Geometry check sheet. Reference: drawing and pictorial views, mm from the part's lowest x, y, z. A direction names the side the tool comes from. Round coordinates to 2 decimals unless told otherwise and drop trailing zeros. Order: outer loops, then holes, each group sorted by start corner. A loop starts at its lowest first (then second) coordinate and runs counter-clockwise, first axis right, second up.
(1) Go/stop test with flat-tipped pins: pin 1 (5 mm diameter, centred on y = 2.5, z = 6, fed in from +X); pin 2 (1.6 mm diameter, centred on x = 7, z = 4.5, fed in from +Y); pin 3 (3 mm diameter, centred on x = 11.5, y = 7, fed in from +Z). Record where each tip stops, or that it passes through.
(2) Sectioned sample at C-C (y = 6.5). Record the boundary of the cut face in (x, z), plus the area to 3 significant figures.
(3) Release check for a two-part mould opening along X. For the marked faces 3, 4 and 5 record: +X half, -X half, draft (parallel to the pull), parting line (faces both ways), or undercut.
(4) Material ranges on line 1 along X through (y, z) = (10.5, 6); line 2 along Y through (x, z) = (7, 6); line 3 along Y through (x, z) = (6.5, 12.5), recorded low to high.
(5) Sectioned sample at B-B (x = 4.75). Record the boundary of the cut face in (y, z).
(6) Sectioned sample at A-A (z = 7). Record the boundary of the cut face in (x, y).
(7) Sectioned sample at D-D (z = 8.75). Record the boundary of the cut face in (x, y), plus the area to 3 significant figures.
(8) Set-up check for the marked faces 1 and 2: record each of +Z, -Z, +X, -X, +Y, -Y from which the full face is reachable in a straight line by a thin tool's end or side.
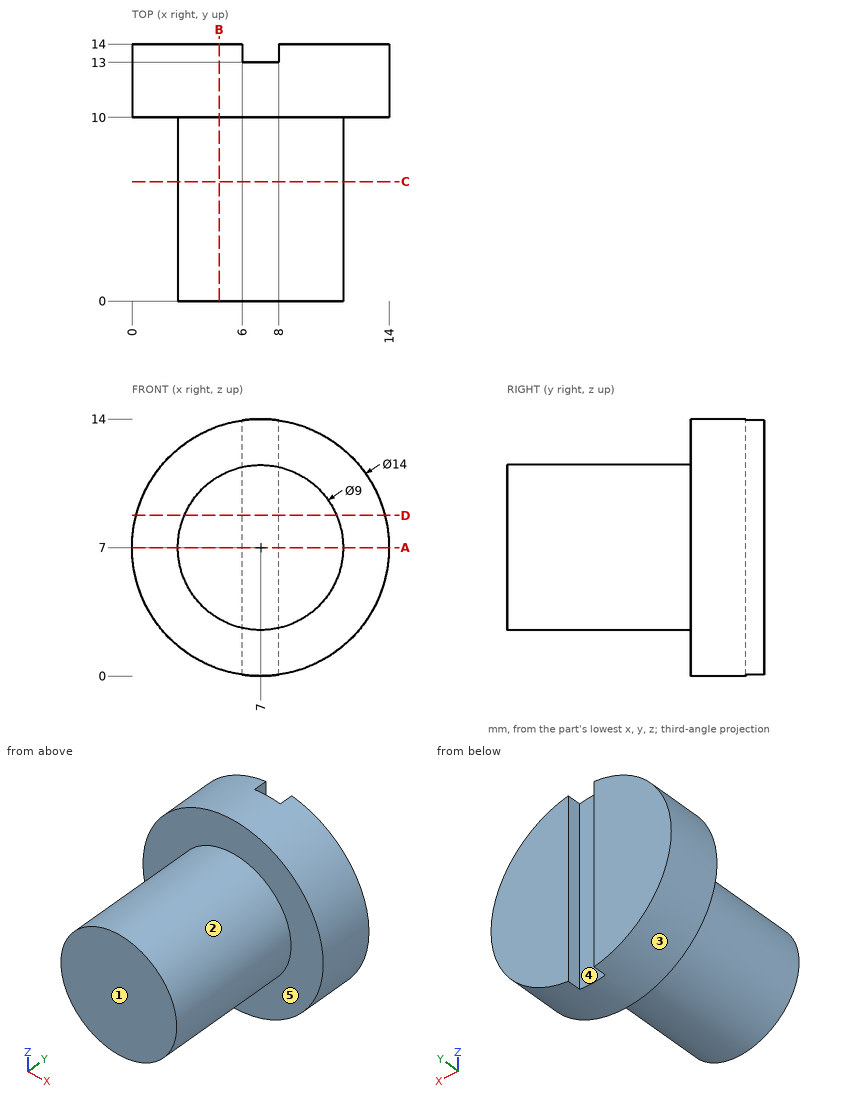
Answer below:
1. pin 1: stops at x = 11.5
1. pin 2: stops at y = 13
1. pin 3: stops at z = 10.35
2. outline: circle Ø9 at (7, 7)
2. area: 63.6 mm2
3. face 3: parting line
3. face 4: undercut
3. face 5: draft
4. line 1: x = 0.07 to 13.93
4. line 2: y = 0 to 13
4. line 3: y = 10 to 13
5. outline: (0, 3.1) - (10, 3.1) - (10, 0.37) - (14, 0.37) - (14, 13.63) - (10, 13.63) - (10, 10.9) - (0, 10.9) - close
6. outline: (0, 10) - (2.5, 10) - (2.5, 0) - (11.5, 0) - (11.5, 10) - (14, 10) - (14, 14) - (8, 14) - (8, 13) - (6, 13) - (6, 14) - (0, 14) - close
7. outline: (0.22, 10) - (2.85, 10) - (2.85, 0) - (11.15, 0) - (11.15, 10) - (13.78, 10) - (13.78, 14) - (8, 14) - (8, 13) - (6, 13) - (6, 14) - (0.22, 14) - close
7. area: 135 mm2
8. face 1: +Z, -Z, +X, -X, -Y
8. face 2: -Y
